For this review, use the dimensioned drawing (mm, ordinates from the lowest corner) and the shaded views. Coordinates: 2 decimals unless noted, no trailing zeros. Loops run counter-clockwise (first coordinate to the right, second up) from the corner with the lowest first, then second, coordinate; pieces in that order, holes last. Notation, with made-up numbers: (-5.75, -1) - (31.25, -1) arc R27 ccw to (31.25, 29) - close; hole circle Ø3 at (36.25, 5). An arc over 180 degrees is marked (long way). Answer in a Markdown table with one row per item. Add a question column.
(1) We need section D-D, the plane x = 4.5. Give the number of separate pieces and of enclosed holes in the cut face, plus the area to 3 significant figures.
(2) To check wall thickness, follow L1, parallel to Y at x = 2, z = 20; L2, parallel to Z at x = 2, y = 153; L3, parallel to Y at x = 1.5, z = 7.5. State the ranges of each line that lie inside material, in increasing order. Write a range as [from, to].
(3) We need section A-A, the plane z = 67.5. Write out the cut boundary in (x, y).
(4) We need section B-B, the plane y = 153. Write out the cut boundary in (x, z), plus the area to 3 significant figures.
(5) We need section C-C, the plane z = 20. Write out the cut boundary in (x, y).
(6) Clearance check with flat-ended pins moving along their axes: pin 1 (1.5 mm diameter, centred on x = 1, z = 61, fed in from -Y); pin 2 (1.9 mm diameter, centred on x = 2.5, z = 42, fed in from -Y); pin 3 (3 mm diameter, centred on x = 3.5, z = 33, fed in from +Y). State where each tip first meets the part, or that it passes through.
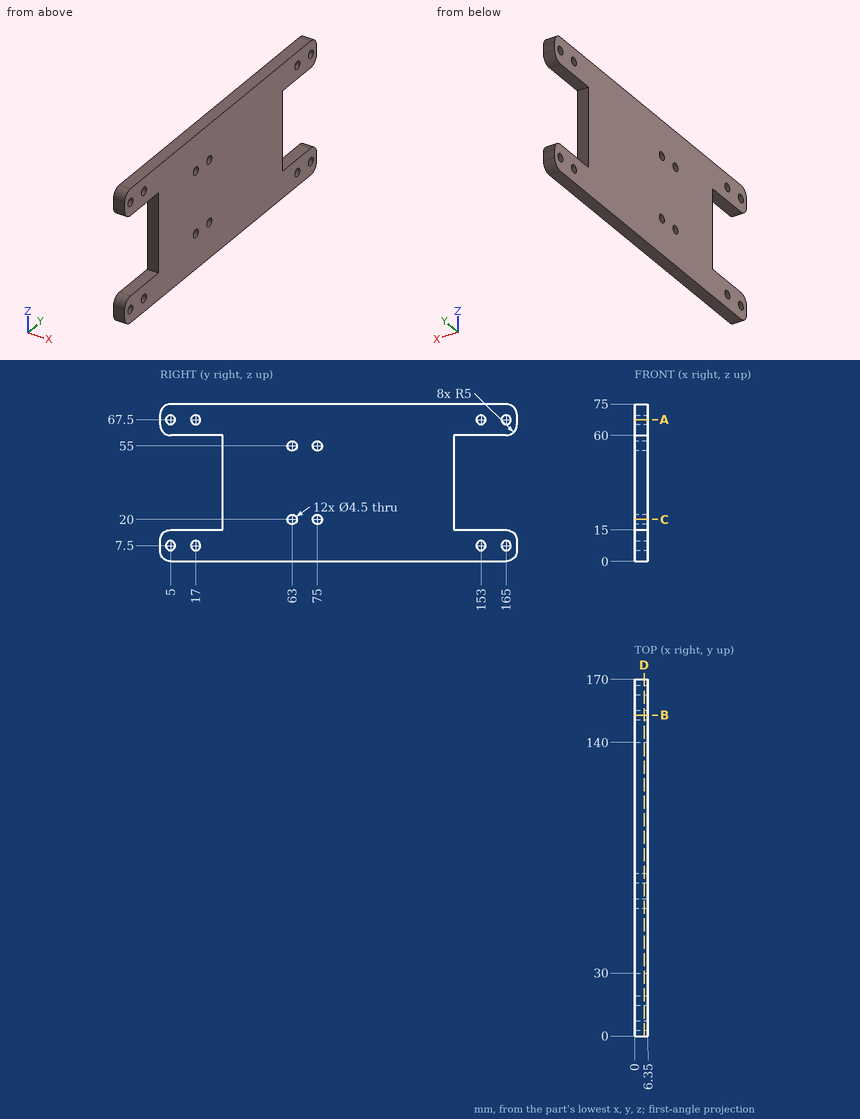
Responses:
| question | item | result |
|---|---|---|
| 1 | separate pieces | 1 |
| 1 | enclosed holes | 12 |
| 1 | area | 9,820 mm2 |
| 2 | L1 | y = [30, 60.75], [65.25, 72.75], [77.25, 140] |
| 2 | L2 | z = [0, 5.25], [9.75, 15], [60, 65.25], [69.75, 75] |
| 2 | L3 | y = [0, 2.75], [7.25, 14.75], [19.25, 150.75], [155.25, 162.75], [167.25, 170] |
| 3 | outline | (0, 0) - (6.35, 0) - (6.35, 2.75) - (0, 2.75) - close; (0, 7.25) - (6.35, 7.25) - (6.35, 14.75) - (0, 14.75) - close; (0, 19.25) - (6.35, 19.25) - (6.35, 150.75) - (0, 150.75) - close; (0, 155.25) - (6.35, 155.25) - (6.35, 162.75) - (0, 162.75) - close; (0, 167.25) - (6.35, 167.25) - (6.35, 170) - (0, 170) - close |
| 4 | outline | (0, 0) - (6.35, 0) - (6.35, 5.25) - (0, 5.25) - close; (0, 9.75) - (6.35, 9.75) - (6.35, 15) - (0, 15) - close; (0, 60) - (6.35, 60) - (6.35, 65.25) - (0, 65.25) - close; (0, 69.75) - (6.35, 69.75) - (6.35, 75) - (0, 75) - close |
| 4 | area | 133 mm2 |
| 5 | outline | (0, 30) - (6.35, 30) - (6.35, 60.75) - (0, 60.75) - close; (0, 65.25) - (6.35, 65.25) - (6.35, 72.75) - (0, 72.75) - close; (0, 77.25) - (6.35, 77.25) - (6.35, 140) - (0, 140) - close |
| 6 | pin 1 | stops at y = 1.2 |
| 6 | pin 2 | stops at y = 30 |
| 6 | pin 3 | stops at y = 140 |
